```python
from build123d import *

# Parameters (mm, degrees)
SKIZZE1_W                       = 330
SKIZZE1_H                       = 156
AUFSATZ_LINEAR_AUSTRAGEN1_DEPTH = 4
SKIZZE2_R                       = 2.25
SKIZZE2_W                       = 31.1
SKIZZE2_H                       = 110
SCHNITT_LINEAR_AUSTRAGEN1_DEPTH = 183.551362635
M3_GEWINDEBOHRUNG1_D            = 2.5
SKIZZE5_R                       = 19
SCHNITT_LINEAR_AUSTRAGEN2_DEPTH = 183.551362635
SKIZZE7_W                       = 35
SKIZZE7_H                       = 25
SCHNITT_LINEAR_AUSTRAGEN3_DEPTH = 183.551362635
VERRUNDUNG1_R                   = 2
SCHNITT_LINEAR_AUSTRAGEN4_DEPTH = 183.551362635
SKIZZE9_W                       = 4
SKIZZE9_H                       = 30
SCHNITT_LINEAR_AUSTRAGEN5_DEPTH = 183.551362635


with BuildPart() as part:
    # Skizze1 → Aufsatz-Linear austragen1 (new body)
    with BuildSketch(Plane.XY):
        Rectangle(SKIZZE1_W, SKIZZE1_H)
    extrude(amount=AUFSATZ_LINEAR_AUSTRAGEN1_DEPTH)

    # Skizze2 → Schnitt-Linear austragen1 (cut, through all)
    with BuildSketch(Plane.XY.offset(4)):
        with Locations((-105.9, 46)):
            Circle(SKIZZE2_R)
        with Locations((-105.9, -46)):
            Circle(SKIZZE2_R)
        with Locations((105.9, -46)):
            Circle(SKIZZE2_R)
        with Locations((105.9, 46)):
            Circle(SKIZZE2_R)
        with Locations((-40, 65)):
            Circle(SKIZZE2_R)
        with Locations((40, 65)):
            Circle(SKIZZE2_R)
        with Locations((-40, -65)):
            Circle(SKIZZE2_R)
        with Locations((40, -65)):
            Circle(SKIZZE2_R)
        with Locations((-135, -65)):
            Circle(SKIZZE2_R)
        with Locations((-135, 65)):
            Circle(SKIZZE2_R)
        with Locations(Location((135, -65, 0), (0, 0, 180))):
            Circle(SKIZZE2_R)
        with Locations(Location((135, 65, 0), (0, 0, 180))):
            Circle(SKIZZE2_R)
        with Locations((133.45, 0)):
            Rectangle(SKIZZE2_W, SKIZZE2_H)
        with Locations((-133.45, 0)):
            Rectangle(SKIZZE2_W, SKIZZE2_H)
    extrude(amount=-SCHNITT_LINEAR_AUSTRAGEN1_DEPTH, mode=Mode.SUBTRACT)

    # M3 Gewindebohrung1 (through all)
    with Locations(Plane.XY.offset(4)):
        with Locations((16, -16), (0, 0), (16, 16), (-16, -16), (-16, 16)):
            Hole(M3_GEWINDEBOHRUNG1_D / 2)

    # Skizze5 → Schnitt-Linear austragen2 (cut, through all)
    with BuildSketch(Plane.XY.offset(4)):
        Circle(SKIZZE5_R)
    extrude(amount=-SCHNITT_LINEAR_AUSTRAGEN2_DEPTH, mode=Mode.SUBTRACT)

    # Skizze7 → Schnitt-Linear austragen3 (cut, through all)
    with BuildSketch(Plane.XY.offset(4)):
        with Locations((0, -42.5)):
            Rectangle(SKIZZE7_W, SKIZZE7_H)
        with Locations((0, 40.787318201)):
            Rectangle(SKIZZE7_W, SKIZZE7_H)
    extrude(amount=-SCHNITT_LINEAR_AUSTRAGEN3_DEPTH, mode=Mode.SUBTRACT)

    # Verrundung1
    verrundung1_edges = [part.edges().sort_by_distance(p)[0] for p in [
        (-17.5, 28.287318201, 2),
        (-17.5, 53.287318201, 2),
        (17.5, 53.287318201, 2),
        (17.5, 28.287318201, 2),
        (17.5, -30, 2),
        (17.5, -55, 2),
        (-17.5, -55, 2),
        (-17.5, -30, 2),
        (149, 55, 2),
        (149, -55, 2),
        (117.9, -55, 2),
        (117.9, 55, 2),
        (-149, -55, 2),
        (-149, 55, 2),
        (-117.9, 55, 2),
        (-117.9, -55, 2),
    ]]
    fillet(verrundung1_edges, radius=VERRUNDUNG1_R)

    # Skizze8 → Schnitt-Linear austragen4 (cut, through all)
    with BuildSketch(Plane.XY.offset(4)):
        with BuildLine():
            Line((-93.9, 9), (-93.9, -9))
            Line((-93.9, -9), (-93.9, -53))
            ThreePointArc((-93.9, -53), (-93.314213562, -54.414213562), (-91.9, -55))
            Line((-91.9, -55), (-55.9, -55))
            ThreePointArc((-55.9, -55), (-54.485786438, -54.414213562), (-53.9, -53))
            Line((-53.9, -53), (-53.9, -9))
            Line((-53.9, -9), (-53.9, 9))
            Line((-53.9, 9), (-53.9, 53))
            ThreePointArc((-53.9, 53), (-54.485786438, 54.414213562), (-55.9, 55))
            Line((-55.9, 55), (-91.9, 55))
            ThreePointArc((-91.9, 55), (-93.314213562, 54.414213562), (-93.9, 53))
            Line((-93.9, 53), (-93.9, 9))
        make_face()
        with BuildLine():
            Line((53.9, 9), (53.9, 53))
            ThreePointArc((53.9, 53), (54.485786438, 54.414213562), (55.9, 55))
            Line((55.9, 55), (91.9, 55))
            ThreePointArc((91.9, 55), (93.314213562, 54.414213562), (93.9, 53))
            Line((93.9, 53), (93.9, 9))
            Line((93.9, 9), (93.9, -9))
            Line((93.9, -9), (93.9, -53))
            ThreePointArc((93.9, -53), (93.314213562, -54.414213562), (91.9, -55))
            Line((91.9, -55), (55.9, -55))
            ThreePointArc((55.9, -55), (54.485786438, -54.414213562), (53.9, -53))
            Line((53.9, -53), (53.9, -9))
            Line((53.9, -9), (53.9, 9))
        make_face()
    extrude(amount=-SCHNITT_LINEAR_AUSTRAGEN4_DEPTH, mode=Mode.SUBTRACT)

    # Skizze9 → Schnitt-Linear austragen5 (cut, through all)
    with BuildSketch(Plane.XY.offset(4)):
        with Locations((-163, 31)):
            Rectangle(SKIZZE9_W, SKIZZE9_H)
        with Locations((-163, -31)):
            Rectangle(SKIZZE9_W, SKIZZE9_H)
        with Locations((163, -31)):
            Rectangle(SKIZZE9_W, SKIZZE9_H)
        with Locations((163, 31)):
            Rectangle(SKIZZE9_W, SKIZZE9_H)
        with Locations((-28, -31)):
            Rectangle(SKIZZE9_W, SKIZZE9_H)
        with Locations((-28, 31)):
            Rectangle(SKIZZE9_W, SKIZZE9_H)
        with Locations((28, -31)):
            Rectangle(SKIZZE9_W, SKIZZE9_H)
        with Locations((28, 31)):
            Rectangle(SKIZZE9_W, SKIZZE9_H)
    extrude(amount=-SCHNITT_LINEAR_AUSTRAGEN5_DEPTH, mode=Mode.SUBTRACT)


solid = part.part
```
Geometry check sheet. Reference: the model listing, model coordinates, mm. Round coordinates to 2 decimals unless told otherwise and drop trailing zeros. Loops run counter-clockwise (first coordinate to the right, second up) from the corner with the lowest first, then second, coordinate; pieces in that order, holes last. Notation, with made-up numbers: (-33.5, 75.5) - (-16.5, 75.5) arc R16 ccw to (-16.5, 85.5) - close; hole circle Ø11 at (-38, 78.25). An arc over 180 degrees is marked (long way). Use a Markdown table: item, result.
Q1. Draft check along Y on faces 1 (the cylindrical face through (8.767, -16.856, 2.028)), 2 (the flat face through (-39, 1, 4)). Enter one of: released by +Y, released by -Y, zero draft, split by the parting line, or undercut.
Solutions:
| item | result |
|---|---|
| face 1 | undercut |
| face 2 | zero draft |
Q2. Material ranges on line 1 (Y direction, x = 135, z = 1.65); line 2 (X direction, y = 51, z = 1); line 3 (Y direction, x = 133, z = 3.6), recorded low to high.
Solutions:
| item | result |
|---|---|
| line 1 | y = -78 to -67.25, -62.75 to -55, 55 to 62.75, 67.25 to 78 |
| line 2 | x = -165 to -149, -117.9 to -93.9, -53.9 to -17.5, 17.5 to 53.9, 93.9 to 117.9, 149 to 165 |
| line 3 | y = -78 to -66.03, -63.97 to -55, 55 to 63.97, 66.03 to 78 |
Q3. Cross-section at B-B on x = 0. Record the cut outline in (y, z), plus the area to 3 significant figures.
Solutions:
| item | result |
|---|---|
| outline | (-78, 0) - (-55, 0) - (-55, 4) - (-78, 4) - close; (-30, 0) - (-19, 0) - (-19, 4) - (-30, 4) - close; (19, 0) - (28.29, 0) - (28.29, 4) - (19, 4) - close; (53.29, 0) - (78, 0) - (78, 4) - (53.29, 4) - close |
| area | 272 mm2 |
Q4. Cross-section at D-D on z = 2.65. State how many separate pieces and enclosed holes the cut face has, plus the area to 3 significant figures.
Solutions:
| item | result |
|---|---|
| separate pieces | 1 |
| enclosed holes | 27 |
| area | 31,800 mm2 |
Q5. Cross-section at C-C on y = 0. Record the cut outline in (x, z), plus the area to 3 significant figures.
Solutions:
| item | result |
|---|---|
| outline | (-165, 0) - (-149, 0) - (-149, 4) - (-165, 4) - close; (-117.9, 0) - (-93.9, 0) - (-93.9, 4) - (-117.9, 4) - close; (-53.9, 0) - (-19, 0) - (-19, 4) - (-53.9, 4) - close; (19, 0) - (53.9, 0) - (53.9, 4) - (19, 4) - close; (93.9, 0) - (117.9, 0) - (117.9, 4) - (93.9, 4) - close; (149, 0) - (165, 0) - (165, 4) - (149, 4) - close |
| area | 599 mm2 |
Q6. Cross-section at A-A on y = -25. Record the cut outline in (x, z), plus the area to 3 significant figures.
Solutions:
| item | result |
|---|---|
| outline | (-161, 0) - (-149, 0) - (-149, 4) - (-161, 4) - close; (-117.9, 0) - (-93.9, 0) - (-93.9, 4) - (-117.9, 4) - close; (-53.9, 0) - (-30, 0) - (-30, 4) - (-53.9, 4) - close; (-26, 0) - (26, 0) - (26, 4) - (-26, 4) - close; (30, 0) - (53.9, 0) - (53.9, 4) - (30, 4) - close; (93.9, 0) - (117.9, 0) - (117.9, 4) - (93.9, 4) - close; (149, 0) - (161, 0) - (161, 4) - (149, 4) - close |
| area | 687 mm2 |
Q7. Go/stop test with flat-tipped pins: P1, Ø2, axis at y = 37, z = 1, coming from the -X side; P2, Ø1, axis at y = -27, z = 1.5, coming from the +X side. Record where each tip stops, or that it passes through.
Solutions:
| item | result |
|---|---|
| P1 | stops at x = -161 |
| P2 | stops at x = 161 |
